Part print with two shaded views. Sizes in mm from the minimum x, y, z corner. A direction names the side the tool comes from. Round coordinates to 2 decimals unless told otherwise and drop trailing zeros. Write each loop counter-clockwise with the first axis right and the second up, starting at its lowest first coordinate (ties: lowest second). Pieces come first, ordered by that corner, then holes. Notation, with made-up numbers: (-19, 16) -> (12, 16) arc R24 ccw to (12, 39) -> close; hole circle Ø8 at (-37.5, 4). An arc over 180 degrees is marked (long way). Put each result on its own line as item: value. Start each with the question number.
1. Saw through at C-C on z = 4. List the corners of the cut face in (x, y).
2. Flat gauge pins, fed straight in: P1, Ø2, axis at x = 3.5, z = 7.5, coming from the +Y side; P2, Ø8, axis at y = 14.5, z = 3, coming from the -X side. Where does each tip first touch, or does it go through?
3. Drill centre lines: line 1 (X direction, y = 11, z = 14.75); line 2 (Y direction, x = 10.25, z = 0.75); line 3 (Y direction, x = 25.6, z = 8). Where is each one in solid material? Low to high. Write a range as from..to.
4. Pull direction Z, two halves, no side cores. Call the marked faces 3 and 4: pulls with the +Z half, pulls with the -Z half, needs draft (parallel to the pull), parting line crosses it, or undercut.
5. Saw through at D-D on x = 24.5. List the corners of the cut face in (y, z).
6. Saw through at B-B on y = 21. List the corners of the cut face in (x, z).
7. Saw through at A-A on z = 8. List the corners of the cut face in (x, y), and give its area (3 significant figures).
8. 3-axis set-ups, long thin cutter, end or side, ignore diameter. For the marked faces 1 and 2: which of +Z, -Z, +X, -X, +Y, -Y reach the whole face in a straight line?
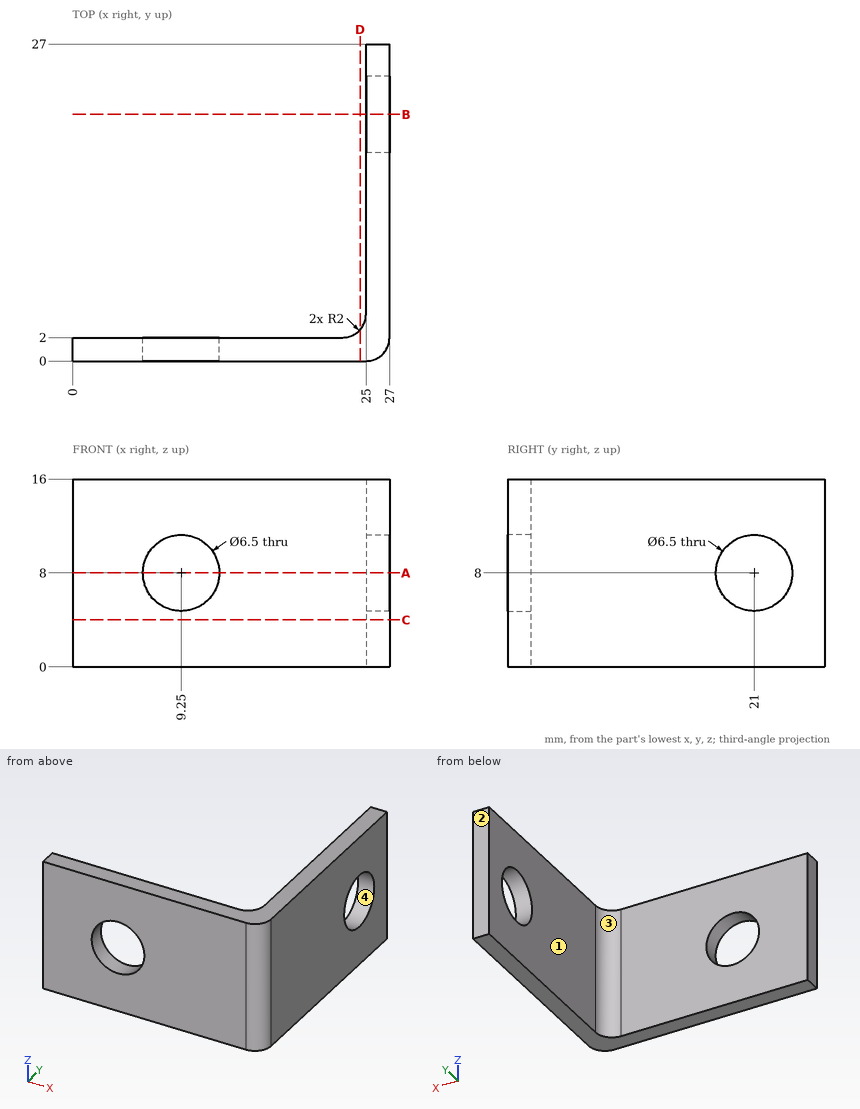
Return value:
1. outline: (0, 0) -> (25, 0) arc R2 ccw to (27, 2) -> (27, 27) -> (25, 27) -> (25, 4) arc R2 cw to (23, 2) -> (0, 2) -> close
2. P1: stops at y = 2
2. P2: stops at x = 25
3. line 1: x = 25..27
3. line 2: y = 0..2
3. line 3: y = 0.09..17.75, 24.25..27
4. face 3: needs draft
4. face 4: undercut
5. outline: (0, 0) -> (2.68, 0) -> (2.68, 16) -> (0, 16) -> close
6. outline: (25, 0) -> (27, 0) -> (27, 4.75) -> (25, 4.75) -> close; (25, 11.25) -> (27, 11.25) -> (27, 16) -> (25, 16) -> close
7. outline: (0, 0) -> (6, 0) -> (6, 2) -> (0, 2) -> close; (12.5, 0) -> (25, 0) arc R2 ccw to (27, 2) -> (27, 17.75) -> (25, 17.75) -> (25, 4) arc R2 cw to (23, 2) -> (12.5, 2) -> close; (25, 24.25) -> (27, 24.25) -> (27, 27) -> (25, 27) -> close
7. area: 78.0 mm^2
8. face 1: +Z, -Z, -X, +Y
8. face 2: +Z, -Z, +X, -X, +Y
